Input: part model. Units: mm. Frame: model coordinates. A direction names the side the tool comes from. Coordinates: 2 decimals unless noted, no trailing zeros. Order: outer loops, then holes, each group sorted by start corner. A loop starts at its lowest first (then second) coordinate and runs counter-clockwise, first axis right, second up.
from build123d import *

# Parameters (mm, degrees)
SKETCH1_R               = 6
BOSS_EXTRUDE3_DEPTH     = 7
SKETCH6_R               = 25
BOSS_EXTRUDE4_DEPTH     = 5
CHAMFER1_SIZE           = 4
SKETCH8_R               = 6
BOSS_EXTRUDE5_DEPTH     = 70
SKETCH9_R               = 3
BOSS_EXTRUDE6_DEPTH     = 2
SKETCH10_R              = 7.5
BOSS_EXTRUDE7_DEPTH     = 5
CHAMFER2_SIZE           = 2
SKETCH13_W              = 30
SKETCH13_H              = 8
CUT_EXTRUDE1_DEPTH      = 66
CUT_EXTRUDE1_DEPTH_BACK = 41.4
FILLET1_R               = 1


with BuildPart() as part:
    # Sketch1 → Boss-Extrude3 (new body, symmetric)
    with BuildSketch(Plane.XY):
        with BuildLine():
            Line((0, 13.4), (-22, 13.4))
            Line((-22, 13.4), (-22, -13.4))
            Line((-22, -13.4), (0, -13.4))
            ThreePointArc((0, -13.4), (13.4, 0), (0, 13.4))
        make_face()
        Circle(SKETCH1_R, mode=Mode.SUBTRACT)
    extrude(amount=BOSS_EXTRUDE3_DEPTH, both=True)

    # Sketch6 → Boss-Extrude4 (add)
    with BuildSketch(Plane.ZY.offset(22)):
        Circle(SKETCH6_R)
    extrude(amount=BOSS_EXTRUDE4_DEPTH)

    # Sketch7 → Cut-Revolve2 (revolve, cut)
    with BuildSketch(Plane.XY):
        Polygon((-27, 0), (-23.5, 0), (-27, -18), align=None)
    revolve(axis=Axis((-27, 0, 0), (1, 0, 0)), mode=Mode.SUBTRACT)

    # Chamfer1
    chamfer1_edges = [part.edges().sort_by_distance(p)[0] for p in [
        (-22, 0, -25),
    ]]
    chamfer(chamfer1_edges, length=CHAMFER1_SIZE)

    # Sketch8 → Boss-Extrude5 (add)
    with BuildSketch(Plane(origin=(-22, 0, 0), x_dir=(0, 0, -1), z_dir=(1, 0, 0))):
        Circle(SKETCH8_R)
    extrude(amount=-BOSS_EXTRUDE5_DEPTH)

    # Sketch9 → Boss-Extrude6 (add)
    with BuildSketch(Plane(origin=(0, 13.4, 0), x_dir=(1, 0, 0), z_dir=(0, 1, 0))):
        with Locations((-11, 0)):
            Circle(SKETCH9_R)
    extrude(amount=BOSS_EXTRUDE6_DEPTH)

    # Sketch10 → Boss-Extrude7 (add)
    with BuildSketch(Plane(origin=(0, 15.4, 0), x_dir=(1, 0, 0), z_dir=(0, 1, 0))):
        with Locations((-11, 0)):
            Circle(SKETCH10_R)
    extrude(amount=BOSS_EXTRUDE7_DEPTH)

    # Chamfer2
    chamfer2_edges = [part.edges().sort_by_distance(p)[0] for p in [
        (-18.5, 20.4, 0),
    ]]
    chamfer(chamfer2_edges, length=CHAMFER2_SIZE)

    # Sketch13 → Cut-Extrude1 (cut, two sides)
    with BuildSketch(Plane.ZY.offset(27)) as cut_extrude1_sk:
        with Locations((25, 0)):
            Rectangle(SKETCH13_W, SKETCH13_H)
    extrude(amount=CUT_EXTRUDE1_DEPTH, mode=Mode.SUBTRACT)
    extrude(cut_extrude1_sk.sketch, amount=-CUT_EXTRUDE1_DEPTH_BACK, mode=Mode.SUBTRACT)

    # Fillet1
    fillet1_edges = [part.edges().sort_by_distance(p)[0] for p in [
        (-6, 0, -7),
        (-6, 0, 7),
        (-22, 0, 7),
        (-11, -13.4, 7),
        (13.4, 0, 7),
        (-11, -13.4, -7),
        (-22, 0, -7),
        (-11, 13.4, -7),
        (13.4, 0, -7),
        (-22, -13.4, 0),
        (-22, 13.4, 0),
        (-11, 13.4, 7),
    ]]
    fillet(fillet1_edges, radius=FILLET1_R)


solid = part.part
Item 1: Draft query along X for faces 5 (the face through (-92, 0, 0)), 6 (the face through (-18.493, 16.879, -0.33)), 7 (the face through (-25, -4, 17)). Return one class per face: pulls with the +X half, pulls with the -X half, needs draft (parallel to the pull), parting line crosses it, or undercut.
Response values:
face 5: pulls with the -X half
face 6: undercut
face 7: needs draft
Item 2: Access query for faces 1 (the face through (-25, 4, 17)), 2 (the face through (-57.862, 1.802, -5.723)), 3 (the face through (-11, 20.4, 0)), 4 (the face through (-11.1, 15.4, 3.2)). Directions: +Z, -Z, +X, -X, +Y, -Y. A direction counts if a zero-diameter tool reaches every point of the face in a straight line with its end or side. Return the directions, or none.
Response values:
face 1: +Z, +X, -X
face 2: -X
face 3: +Z, -Z, +X, +Y
face 4: none
Item 3: Ray query, probe 1 along Y at (x, z) = (0, -2.75); probe 2 along Y at (x, z) = (-6.5, -3); probe 3 along Z at (x, y) = (2, -11.5). Return the intervals inside material, ascending.
Response values:
probe 1: y = -13.4 to -6, 6 to 13.4
probe 2: y = -13.4 to 13.4, 15.4 to 20.4
probe 3: z = -7 to 7
Item 4: Pin query (flat end, axial travel): pin 1 Ø4 at (x, y) = (-24.5, 1) entering from +Z; pin 2 Ø7 at (x, y) = (0, 0) entering from +Z; pin 3 Ø13 at (x, z) = (-8, 0) entering from +Y; pin 4 Ø2 at (y, z) = (-17, 8.5) entering from -X. Return the tip coordinate at first contact, or that it passes through.
Response values:
pin 1: stops at z = 10
pin 2: passes through
pin 3: stops at y = 20.4
pin 4: stops at x = -27
Item 5: Cut plane C-C on x = -11. Return loops of the section in (y, z), then the cut area to 3 significant figures.
Response values:
outline: (-13.4, -6) arc R1 ccw to (-12.4, -7) - (12.4, -7) arc R1 ccw to (13.4, -6) - (13.4, -3) - (15.4, -3) - (15.4, -7.5) - (18.4, -7.5) - (20.4, -5.5) - (20.4, 5.5) - (18.4, 7.5) - (15.4, 7.5) - (15.4, 3) - (13.4, 3) - (13.4, 6) arc R1 ccw to (12.4, 7) - (-12.4, 7) arc R1 ccw to (-13.4, 6) - close
area: 457 mm2
Item 6: Cut plane D-D on x = -60. Return loops of the section in (y, z), then the cut area to 3 significant figures.
Response values:
outline: circle Ø12 at (0, 0)
area: 113 mm2
Item 7: Cut plane B-B on y = 0. Return loops of the section in (x, z), then the cut area to 3 significant figures.
Response values:
outline: (-92, -6) - (-24.67, -6) - (-27, -18) - (-27, -25) - (-26, -25) - (-22, -21) - (-22, -8) arc R1 cw to (-21, -7) - (-7, -7) arc R1 ccw to (-6, -6) - (-6, 6) arc R1 ccw to (-7, 7) - (-21, 7) arc R1 cw to (-22, 8) - (-22, 10) - (-25.44, 10) - (-24.67, 6) - (-92, 6) - close; (6, -6) arc R1 ccw to (7, -7) - (12.4, -7) arc R1 ccw to (13.4, -6) - (13.4, 6) arc R1 ccw to (12.4, 7) - (7, 7) arc R1 ccw to (6, 6) - close
area: 1,250 mm2
